```python
from build123d import *

# Parameters (mm, degrees)
BOSS_EXTRUDE1_DEPTH  = 19
BOSS_EXTRUDE2_DEPTH  = 3.5
BOSS_EXTRUDE3_DEPTH  = 3.5
SKETCH4_W            = 114.479344172
SKETCH4_H            = 30
BOSS_EXTRUDE4_DEPTH  = 25
CUT_EXTRUDE1_DEPTH   = 25
FILLET1_R            = 2.5
BOSS_EXTRUDE8_DEPTH  = 19
BOSS_EXTRUDE9_DEPTH  = 3.5
BOSS_EXTRUDE10_DEPTH = 3.5
CUT_EXTRUDE2_DEPTH   = 43.5
FILLET2_R            = 2.5
SKETCH13_W           = 6.5
SKETCH13_H           = 11.5
CUT_EXTRUDE4_DEPTH   = 172.520091892
SKETCH14_W           = 35.5
SKETCH14_H           = 6
CUT_EXTRUDE5_DEPTH   = 1.5


with BuildPart() as part:
    # Sketch1 → Boss-Extrude1 (new body)
    with BuildSketch(Plane(origin=(0, 0, 0), x_dir=(1, 0, 0), z_dir=(0, 1, 0))):
        Polygon((0, 0), (140, 0), (140, 10), (114.5, 35.5), (0, 35.5), align=None)
    extrude(amount=BOSS_EXTRUDE1_DEPTH)

    # Sketch2 → Boss-Extrude2 (add)
    with BuildSketch(Plane(origin=(0, 19, 0), x_dir=(1, 0, 0), z_dir=(0, 1, 0))):
        Polygon((140, 0), (105, 0), (105, 17), (133, 17), (140, 10), align=None)
    extrude(amount=BOSS_EXTRUDE2_DEPTH)

    # Sketch3 → Boss-Extrude3 (add)
    with BuildSketch(Plane.XZ):
        Polygon((140, -10), (133, -17), (105, -17), (105, 0), (140, 0), align=None)
    extrude(amount=BOSS_EXTRUDE3_DEPTH)

    # Sketch4 → Boss-Extrude4 (add)
    with BuildSketch(Plane(origin=(0, 0, -35.5), x_dir=(-1, 0, 0), z_dir=(0, 0, -1))):
        with Locations((-57.25, 9.5)):
            Rectangle(SKETCH4_W, SKETCH4_H)
    extrude(amount=BOSS_EXTRUDE4_DEPTH)

    # Sketch5 → Cut-Extrude1 (cut)
    with BuildSketch(Plane(origin=(0, 19, 0), x_dir=(1, 0, 0), z_dir=(0, 1, 0))):
        with BuildLine():
            Line((30.5, 23), (81.5, 23))
            ThreePointArc((81.5, 23), (87, 17.5), (81.5, 12))
            Line((81.5, 12), (30.5, 12))
            ThreePointArc((30.5, 12), (25, 17.5), (30.5, 23))
        make_face()
    extrude(amount=-CUT_EXTRUDE1_DEPTH, mode=Mode.SUBTRACT)

    # Fillet1
    fillet1_edges = [part.edges().sort_by_distance(p)[0] for p in [
        (56, 0, -12),
        (87, 0, -17.5),
        (56, 0, -23),
        (25, 0, -17.5),
        (25, 19, -17.5),
        (56, 19, -12),
        (87, 19, -17.5),
        (56, 19, -23),
    ]]
    fillet(fillet1_edges, radius=FILLET1_R)

    # Sketch7 → Boss-Extrude8 (add)
    with BuildSketch(Plane(origin=(0, 0, 0), x_dir=(1, 0, 0), z_dir=(0, 1, 0))):
        Polygon((0.010327914, 60.5), (0.010327914, 96), (140.010327914, 96), (140.010327914, 86), (114.510327914, 60.5), align=None)
    extrude(amount=BOSS_EXTRUDE8_DEPTH)

    # Sketch10 → Boss-Extrude9 (add)
    with BuildSketch(Plane(origin=(0, 19, 0), x_dir=(1, 0, 0), z_dir=(0, 1, 0))):
        Polygon((140.010327914, 86), (133.010327914, 79), (105.010327914, 79), (105.010327914, 96), (140.010327914, 96), align=None)
    extrude(amount=BOSS_EXTRUDE9_DEPTH)

    # Sketch11 → Boss-Extrude10 (add)
    with BuildSketch(Plane.XZ):
        Polygon((133.010327914, -79), (140.010327914, -86), (140.010327914, -96), (105.010327914, -96), (105.010327914, -79), align=None)
    extrude(amount=BOSS_EXTRUDE10_DEPTH)

    # Sketch12 → Cut-Extrude2 (cut)
    with BuildSketch(Plane.XZ):
        with BuildLine():
            Line((30.510327914, -73), (81.510327914, -73))
            ThreePointArc((81.510327914, -73), (87.010327914, -78.5), (81.510327914, -84))
            Line((81.510327914, -84), (30.510327914, -84))
            ThreePointArc((30.510327914, -84), (25.010327914, -78.5), (30.510327914, -73))
        make_face()
    extrude(amount=-CUT_EXTRUDE2_DEPTH, mode=Mode.SUBTRACT)

    # Fillet2
    fillet2_edges = [part.edges().sort_by_distance(p)[0] for p in [
        (56.010327914, 19, -84),
        (87.010327914, 19, -78.5),
        (56.010327914, 19, -73),
        (25.010327914, 19, -78.5),
        (25.010327914, 0, -78.5),
        (56.010327914, 0, -84),
        (87.010327914, 0, -78.5),
        (56.010327914, 0, -73),
    ]]
    fillet(fillet2_edges, radius=FILLET2_R)

    # Sketch13 → Cut-Extrude4 (cut, through all)
    with BuildSketch(Plane.XY):
        with Locations((3.260327914, 0.25)):
            Rectangle(SKETCH13_W, SKETCH13_H)
    extrude(amount=-CUT_EXTRUDE4_DEPTH, mode=Mode.SUBTRACT)

    # Sketch14 → Cut-Extrude5 (cut)
    with BuildSketch(Plane.ZY):
        with Locations((-17.75, 3)):
            Rectangle(SKETCH14_W, SKETCH14_H)
    extrude(amount=-CUT_EXTRUDE5_DEPTH, mode=Mode.SUBTRACT)


solid = part.part
```
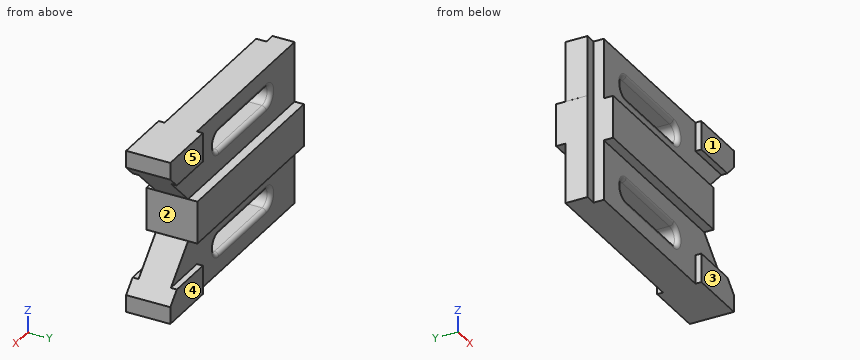
The listing builds one solid part. Answer for the finished solid, in the listing's coordinates (mm). Face numbers are marked on the shaded views. A direction names the side the tool comes from. Coordinates: 2 decimals unless noted, no trailing zeros. Write each loop counter-clockwise with the first axis right and the second up, starting at its lowest first coordinate (ties: lowest second). Pieces come first, ordered by that corner, then holes. Notation, with made-up numbers: M 5.25,-29.75 L 61.25,-29.75 A19 ccw 61.25,3.25 Z; hole C -4,9.25 d3. An arc over 180 degrees is marked long. Use a Markdown table: item, result. Add a question column.
1. Which of the six approach directions +Z, -Z, +X, -X, +Y, -Y give full straight-line access (tool end or side, diameter ignored) to the marked faces 1, 2, 3, 4 and 5?
2. Section D-D (x = 128) is taken. Give the vertices of the cut face in (y, z).
3. Straight lines are drawn through the part: line 1 along Z through (x, y) = (72.5, 5); line 2 along Y through (x, z) = (46, -7); line 3 along Z through (x, y) = (19, -3.25). For each, find the intervals that lie inside material, in ascending order. Write a range as [from, to].
4. Section B-B (x = 51.5) is taken. Give the vertices of the cut face in (y, z).
5. Section C-C (y = 15) is taken. Count the separate pieces of the cut face and the enclosed holes in it, plus the area to 3 significant figures.
6. Given P1, Ø10, axis at y = 16.5, z = -49, coming from the -X side; P2, Ø5, axis at y = -1, z = -36.5, coming from the -X side; P3, Ø8.5, axis at x = 116, z = -9.5, coming from the +Y side, each flat-ended and moving along its own axis, determine where each tip first touches the part or whether it passes through.
7. Section A-A (y = -1.75) is taken. Give the vertices of the cut face in (x, z).
Data:
| question | item | result |
|---|---|---|
| 1 | face 1 | +Z, +X, -X, -Y |
| 1 | face 2 | +X, +Y, -Y |
| 1 | face 3 | -Z, +X, -X, -Y |
| 1 | face 4 | -Z, +X, -X, +Y |
| 1 | face 5 | +Z, +X, -X, +Y |
| 2 | outline | M -3.5,-96 L 22.5,-96 L 22.5,-79 L 19,-79 L 19,-73.99 L 0,-73.99 L 0,-79 L -3.5,-79 Z; M -3.5,-17 L 0,-17 L 0,-22 L 19,-22 L 19,-17 L 22.5,-17 L 22.5,0 L -3.5,0 Z |
| 3 | line 1 | z = [-96, -84], [-73, -23], [-12, 0] |
| 3 | line 2 | y = [0, 19] |
| 3 | line 3 | z = [-60.5, -35.5] |
| 4 | outline | M -5.5,-60.5 L 0,-60.5 L 0,-70.5 A2.5 ccw 2.5,-73 L 16.5,-73 A2.5 ccw 19,-70.5 L 19,-60.5 L 24.5,-60.5 L 24.5,-35.5 L 19,-35.5 L 19,-25.5 A2.5 ccw 16.5,-23 L 2.5,-23 A2.5 ccw 0,-25.5 L 0,-35.5 L -5.5,-35.5 Z; M 0,-96 L 19,-96 L 19,-86.5 A2.5 ccw 16.5,-84 L 2.5,-84 A2.5 ccw 0,-86.5 Z; M 0,-9.5 A2.5 ccw 2.5,-12 L 16.5,-12 A2.5 ccw 19,-9.5 L 19,0 L 0,0 Z |
| 5 | separate pieces | 1 |
| 5 | enclosed holes | 2 |
| 5 | area | 10,800 mm2 |
| 6 | P1 | stops at x = 0.01 |
| 6 | P2 | stops at x = 6.51 |
| 6 | P3 | stops at y = 22.5 |
| 7 | outline | M 6.51,-60.5 L 114.49,-60.5 L 114.49,-35.5 L 6.51,-35.5 Z; M 105,-17 L 133,-17 L 140,-10 L 140,0 L 105,0 Z; M 105.01,-96 L 140.01,-96 L 140.01,-86 L 133.01,-79 L 105.01,-79 Z |
